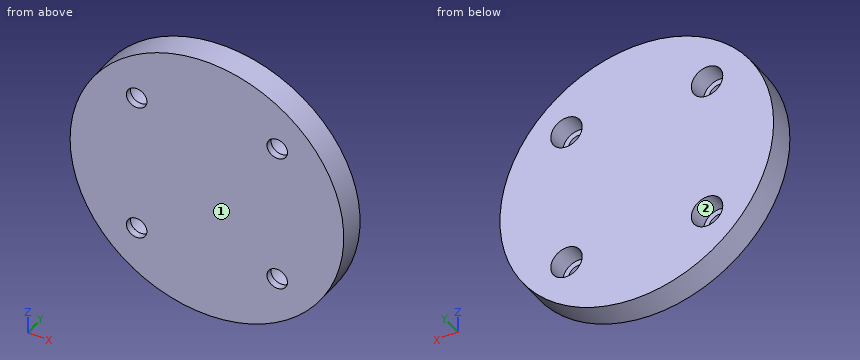
Autodesk Inventor part; units mm, degrees
ref_plane "YZ Plane" through (0, 0, 0) normal (1, 0, 0) x (0, 1, 0)
ref_plane "XZ Plane" through (0, 0, 0) normal (0, 1, 0) x (-1, 0, 0)
ref_plane "XY Plane" through (0, 0, 0) normal (0, 0, 1) x (1, 0, 0)
sketch "Sketch1" plane through (0, 0, 0) normal (0, 1, 0) x (-1, 0, 0)
  circle A0 centre (0, 0) radius 25
  dimension "d0" = 50
extrude "Extrusion1" add sketch "Sketch1" along normal blind 5
sketch "Sketch3" plane through (0, 5, 0) normal (0, 1, 0) x (1, 0, 0)
  point P0 (0, 0)
  point P1 (-12.842, -12.842)
  dimension "d25" = 12.842
  dimension "d26" = 12.842
hole "Hole2" at (-12.842, 5, 12.842) direction (0, -1, 0) diameter 3.75 depth 14.944 counterbore diameter 5.75 counterbore depth 3.75
pattern_circular "Circular Pattern1" count 4 over 360 about axis through (0, -10, 0) along (0, 1, 0) of "Hole2"
properties part number "PrismCageAdapter"
Can you work these out from the model? Positions are in its coordinate system, mm. Face numbers are marked on the shaded views. A direction names the side the tool comes from. Coordinates: 2 decimals unless noted, no trailing zeros. Loops run counter-clockwise (first coordinate to the right, second up) from the corner with the lowest first, then second, coordinate; pieces in that order, holes last. Notation, with made-up numbers: M -27,-24 L -5,-24 A14 cw -5,3 Z; hole C 11.25,-38 d7. An arc over 180 degrees is marked long. Return JSON: item names as keys, results as strings. Group by question number.
Item 1: Imagine slicing it at B-B (x = 21.5). Please give me the cut outline in (y, z).
Item 2: On a 3-axis mill with a long thin cutter (end or side, diameter ignored), from which of +Z, -Z, +X, -X, +Y, -Y can I reach the whole of each face in a straight line? I mean the marked faces 1 and 2. Say none if no direction works.
Item 3: If I drill on L1, parallel to X at y = 3.85, z = 11.5; L2, parallel to Z at x = -15, y = 4.45; L3, parallel to X at y = 3.25, z = 0.5 (3 decimals), over which ranges is the centre line in solid material (lowest first)? Write a range as from..to.
Item 4: I'm going to push flat-ended pins straight in: pin 1 Ø1.5 at (y, z) = (1, 1.5) entering from -X; pin 2 Ø1.7 at (x, z) = (11.5, -12) entering from +Y; pin 3 Ø1 at (x, y) = (13.5, 4) entering from -Z. Where does each tip first touch, or does it pass through?
Item 5: Imagine slicing it at A-A (z = 17). Please give me the cut outline in (x, y).
Verdict:
{
 "1": {"outline": "M 0,-12.76 L 5,-12.76 L 5,12.76 L 0,12.76 Z"},
 "2": {"face 1": "+Z, -Z, +X, -X, -Y", "face 2": "+Y"},
 "3": {"L1": "x = -22.2..-15.38, -10.3..10.3, 15.38..22.2", "L2": "z = -20..-14.74, -10.94..10.94, 14.74..20", "L3": "x = -24.995..24.995"},
 "4": {"pin 1": "stops at x = -24.99", "pin 2": "stops at y = 1.25", "pin 3": "stops at z = -21.35"},
 "5": {"outline": "M -18.33,0 L 18.33,0 L 18.33,5 L -18.33,5 Z"}
}
